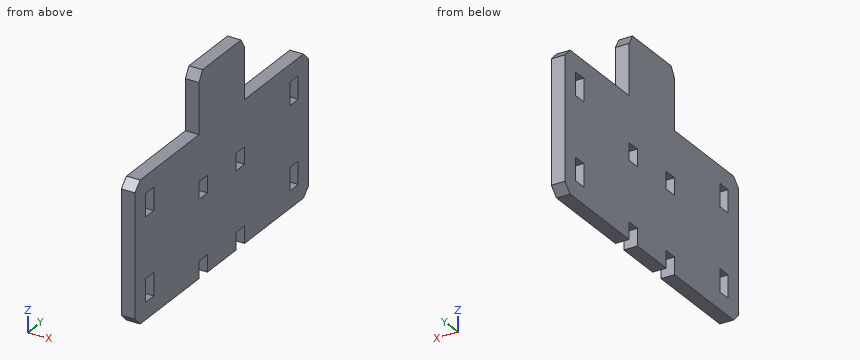
from build123d import *

# Parameters (mm, degrees)
SKETCH1_W           = 10.16
SKETCH1_H           = 6.096
SKETCH1_W_2         = 7.62
BOSS_EXTRUDE1_DEPTH = 3.048
CHAMFER2_SIZE       = 3.81


with BuildPart() as part:
    # Sketch1 → Boss-Extrude1 (new body, symmetric)
    with BuildSketch(Plane(origin=(0, 0, 0), x_dir=(0, 0, -1), z_dir=(1, 0, 0))):
        Polygon((45.72, -63.246), (45.72, -16.5735), (38.1, -16.5735), (38.1, -10.4775), (45.72, -10.4775), (45.72, 10.4775), (38.1, 10.4775), (38.1, 16.5735), (45.72, 16.5735), (45.72, 63.246), (-16.571856626, 63.246), (-16.571856626, 16.5735), (-39.096447575, 16.5735), (-43.495856626, 14.0335), (-43.495856626, -14.0335), (-39.096447575, -16.5735), (-16.571856626, -16.5735), (-16.571856626, -63.246), align=None)
        with Locations((33.02, -52.578)):
            Rectangle(SKETCH1_W, SKETCH1_H, mode=Mode.SUBTRACT)
        with Locations((33.02, 52.578)):
            Rectangle(SKETCH1_W, SKETCH1_H, mode=Mode.SUBTRACT)
        with Locations((-3.871856626, 52.578)):
            Rectangle(SKETCH1_W, SKETCH1_H, mode=Mode.SUBTRACT)
        with Locations((-3.871856626, -52.578)):
            Rectangle(SKETCH1_W, SKETCH1_H, mode=Mode.SUBTRACT)
        with Locations((7.62, 13.5255)):
            Rectangle(SKETCH1_W_2, SKETCH1_H, mode=Mode.SUBTRACT)
        with Locations((7.62, -13.5255)):
            Rectangle(SKETCH1_W_2, SKETCH1_H, mode=Mode.SUBTRACT)
    extrude(amount=BOSS_EXTRUDE1_DEPTH, both=True)

    # Chamfer2
    chamfer2_edges = [part.edges().sort_by_distance(p)[0] for p in [
        (0, -63.246, -45.72),
        (0, -63.246, 16.571856626),
        (0, 63.246, 16.571856626),
        (0, 63.246, -45.72),
    ]]
    chamfer(chamfer2_edges, length=CHAMFER2_SIZE)


solid = part.part
CAD build for the part. Positions are in the model's coordinates, mm. Coordinates: 2 decimals unless noted, no trailing zeros. Loops run counter-clockwise (first coordinate to the right, second up) from the corner with the lowest first, then second, coordinate; pieces in that order, holes last. Notation, with made-up numbers: (55.5, 0) - (113.5, 0) arc R17 cw to (113.5, 7) - close; hole circle Ø8 at (-22, 67). An arc over 180 degrees is marked (long way). Write item = value, one per line. Start each with the question number.
Q1. Cut at B-B, the plane y = -12. List the corners of the cut face in (x, z), then the cut area to 3 significant figures.
Q2. Cut at D-D, the plane z = 26.5. List the corners of the cut face in (x, y), then the cut area to 3 significant figures.
Q3. Drill centre lines: L1, parallel to Y at x = 2, z = -33; L2, parallel to Z at x = -0.5, y = -54.5; L3, parallel to Y at x = 1.25, z = -8. Where is each one in solid material? Low to high.
Q4. Cut at C-C, the plane x = -0.75. Give the number of separate pieces and of enclosed holes in the cut face, then the cut area to 3 significant figures.
Q5. Cut at A-A, the plane y = 53.5. List the corners of the cut face in (x, z), then the cut area to 3 significant figures.
Q6. Flat gauge pins, fed straight in: pin 1 Ø3 at (x, y) = (-1, -14) entering from -Z; pin 2 Ø3 at (x, y) = (-1.5, -53) entering from +Z; pin 3 Ø3 at (x, z) = (1, 20) entering from +Y. Where does each tip first touch, or does it go through?
Computed:
q1.outline = (-3.05, -38.1) - (3.05, -38.1) - (3.05, -11.43) - (-3.05, -11.43) - close; (-3.05, -3.81) - (3.05, -3.81) - (3.05, 43.5) - (-3.05, 43.5) - close
q1.area = 451 mm²
q2.outline = (-3.05, -16.57) - (3.05, -16.57) - (3.05, 16.57) - (-3.05, 16.57) - close
q2.area = 202 mm²
q3.L1 = -63.25 to -55.63, -49.53 to 49.53, 55.63 to 63.25
q3.L2 = -45.72 to -38.1, -27.94 to -1.21, 8.95 to 16.57
q3.L3 = -63.25 to -16.57, -10.48 to 10.48, 16.57 to 63.25
q4.separate_pieces = 1
q4.enclosed_holes = 6
q4.area = 8,300 mm²
q5.outline = (-3.05, -45.72) - (3.05, -45.72) - (3.05, -38.1) - (-3.05, -38.1) - close; (-3.05, -27.94) - (3.05, -27.94) - (3.05, -1.21) - (-3.05, -1.21) - close; (-3.05, 8.95) - (3.05, 8.95) - (3.05, 16.57) - (-3.05, 16.57) - close
q5.area = 256 mm²
q6.pin_1 = -38.1
q6.pin_2 = 16.57
q6.pin_3 = 16.57
